Can you work these out from the model? Positions are in its coordinate system, mm. Face numbers are marked on the shaded views. Round coordinates to 2 decimals unless told otherwise and drop trailing zeros. Loops run counter-clockwise (first coordinate to the right, second up) from the corner with the lowest first, then second, coordinate; pieces in that order, holes last. Notation, with made-up numbers: (40, -17.5) -> (48, -17.5) arc R24 ccw to (48, 20.5) -> close; hole circle Ø10 at (53.5, -14.5). An arc over 180 degrees is marked (long way). Answer as a JSON object with one key per item and string values.
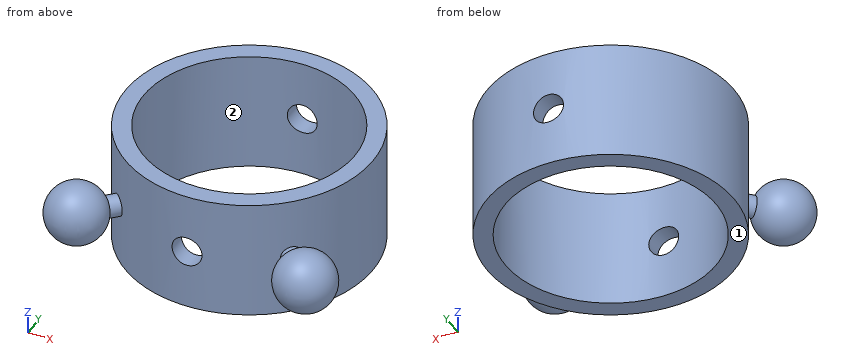
```python
from build123d import *

# Parameters (mm, degrees)
SKETCH1_R               = 20.5
SKETCH1_R_2             = 17.5
BOSS_EXTRUDE1_DEPTH     = 20
SKETCH2_R               = 2.5
CUT_EXTRUDE1_DEPTH      = 21.5
CUT_EXTRUDE1_DEPTH_BACK = 21.5


with BuildPart() as part:
    # Sketch1 → Boss-Extrude1 (new body)
    with BuildSketch(Plane.XY):
        Circle(SKETCH1_R)
        Circle(SKETCH1_R_2, mode=Mode.SUBTRACT)
    extrude(amount=BOSS_EXTRUDE1_DEPTH)

    # Sketch2 → Cut-Extrude1 (cut, two sides)
    with BuildSketch(Plane(origin=(0, 0, 0), x_dir=(1, 0, 0), z_dir=(0, 1, 0))) as cut_extrude1_sk:
        with Locations((0, -10)):
            Circle(SKETCH2_R)
    extrude(amount=CUT_EXTRUDE1_DEPTH, mode=Mode.SUBTRACT)
    extrude(cut_extrude1_sk.sketch, amount=-CUT_EXTRUDE1_DEPTH_BACK, mode=Mode.SUBTRACT)

    # Sketch4 → Revolve1 (revolve)
    with BuildSketch(Plane(origin=(0, 0, 10), x_dir=(-1, 0, 0), z_dir=(0, 0, -1))):
        with BuildLine():
            Line((14.142135624, -14.142135624), (22.627416998, -22.627416998))
            ThreePointArc((22.627416998, -22.627416998), (16.241444529, -23.199802273), (14.5425359, -17.017409634))
            Line((14.5425359, -17.017409634), (12.904698757, -15.379572491))
            Line((12.904698757, -15.379572491), (14.142135624, -14.142135624))
        make_face()
    revolve1 = revolve(axis=Axis((-14.142135624, -14.142135624, 10), (-0.707106781, -0.707106781, 0)))

    # Mirror1: Revolve1 across plane
    add(revolve1.mirror(Plane(origin=(0, 0, 0), x_dir=(0, 0, 1), z_dir=(1, 0, 0))))


solid = part.part
```
Q1. I want a section at D-D, the plane z = 10. Write out the boundary of the cut face in (x, y), then the cut area to 3 significant figures.
Determined:
{"outline": "(-17.02, -14.54) arc R5 ccw (long way) to (-14.54, -17.02) -> (-13.21, -15.68) arc R20.5 ccw to (-2.5, -20.35) -> (-2.5, -17.32) arc R17.5 cw to (-2.5, 17.32) -> (-2.5, 20.35) arc R20.5 ccw to (-15.68, -13.21) -> close; (2.5, -20.35) arc R20.5 ccw to (13.21, -15.68) -> (14.54, -17.02) arc R5 ccw (long way) to (17.02, -14.54) -> (15.68, -13.21) arc R20.5 ccw to (2.5, 20.35) -> (2.5, 17.32) arc R17.5 cw to (2.5, -17.32) -> close", "area": "497 mm²"}
Q2. I'm going to push flat-ended pins straight in: pin 1 (4 mm diameter, centred on y = -2, z = 14.5, fed in from +X); pin 2 (3 mm diameter, centred on x = 18, z = 11.5, fed in from -Y); pin 3 (4 mm diameter, centred on x = -0.5, z = 3, fed in from -Y). Where does each tip first touch, or does it pass through?
Determined:
{"pin 1": "x = 20.5", "pin 2": "y = -24.08", "pin 3": "y = -20.5"}
Q3. I want a section at C-C, the plane x = -10.5. Write out the boundary of the cut face in (y, z), then the cut area to 3 significant figures.
Determined:
{"outline": "(-17.61, 0) -> (-14, 0) -> (-14, 20) -> (-17.61, 20) -> close; (14, 0) -> (17.61, 0) -> (17.61, 20) -> (14, 20) -> close", "area": "144 mm²"}
Q4. We'd pull the mould along X, two halves only. Please class the marked faces 1 and 2: pulls with the +X half, pulls with the -X half, needs draft (parallel to the pull), parting line crosses it, or undercut.
Determined:
{"face 1": "needs draft", "face 2": "undercut"}
Q5. If I drill on L1, parallel to Z at x = 0, y = -19.45; L2, parallel to Y at x = 0, z = 13.5; L3, parallel to X at y = -18.7, z = 10, over which ranges is the centre line in solid material (lowest first)? Write a range as [from, to].
Determined:
{"L1": "[0, 7.5], [12.5, 20]", "L2": "[-20.5, -17.5], [17.5, 20.5]", "L3": "[-24.08, -14.11], [-8.4, -2.5], [2.5, 8.4], [14.11, 24.08]"}
Q6. I want a section at A-A, the plane x = 0. Write out the boundary of the cut face in (y, z), then the cut area to 3 significant figures.
Determined:
{"outline": "(-20.5, 0) -> (-17.5, 0) -> (-17.5, 7.5) -> (-20.5, 7.5) -> close; (-20.5, 12.5) -> (-17.5, 12.5) -> (-17.5, 20) -> (-20.5, 20) -> close; (17.5, 0) -> (20.5, 0) -> (20.5, 7.5) -> (17.5, 7.5) -> close; (17.5, 12.5) -> (20.5, 12.5) -> (20.5, 20) -> (17.5, 20) -> close", "area": "90.0 mm²"}
Q7. I want a section at B-B, the plane y = 0. Write out the boundary of the cut face in (x, z), then the cut area to 3 significant figures.
Determined:
{"outline": "(-20.5, 0) -> (-17.5, 0) -> (-17.5, 20) -> (-20.5, 20) -> close; (17.5, 0) -> (20.5, 0) -> (20.5, 20) -> (17.5, 20) -> close", "area": "120 mm²"}
